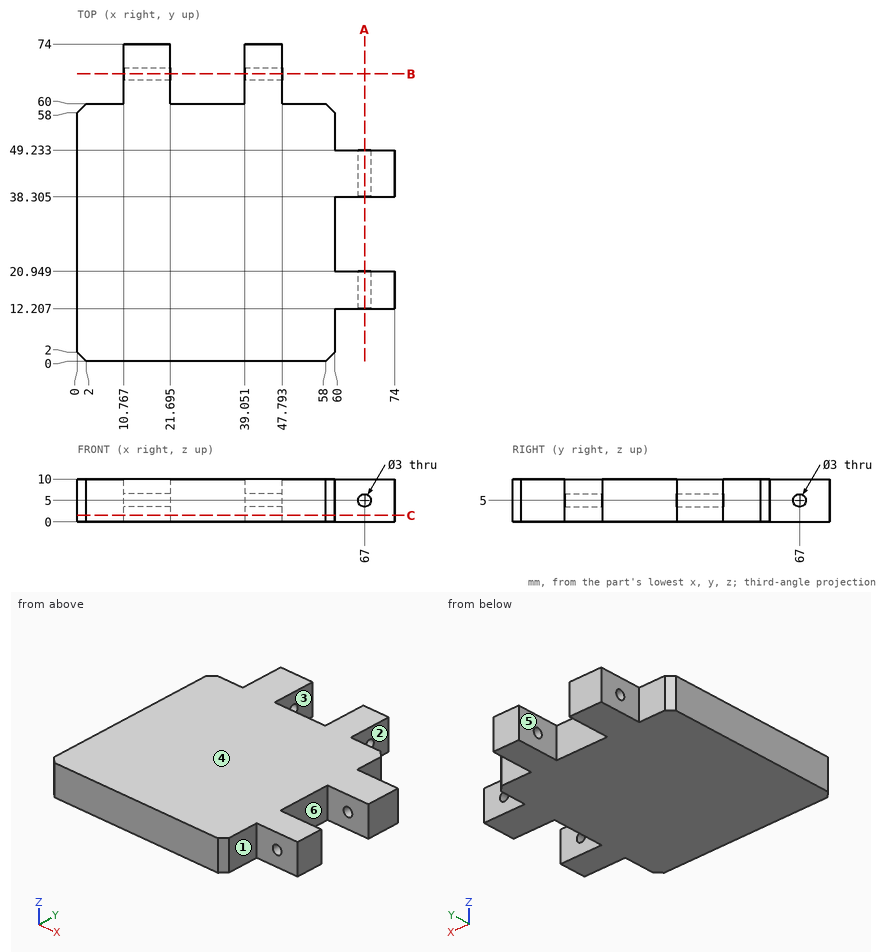
Input: dimensioned drawing with shaded views. Units: mm. Origin: part minimum x, y, z. A direction names the side the tool comes from. Coordinates: 2 decimals unless noted, no trailing zeros. Write each loop counter-clockwise with the first axis right and the second up, starting at its lowest first coordinate (ties: lowest second). Pieces come first, ordered by that corner, then holes. Notation, with made-up numbers: M 60,-8 L 101,-8 A26 ccw 101,30 Z; hole C 21,26 d7. An arc over 180 degrees is marked long. Answer as a JSON object with one key per item and string values. Group by question number.
(1) Ray query, line 1 along X through (y, z) = (44.25, 5); line 2 along Z through (x, y) = (67, 43). Return the intervals inside material, ascending. Write a range as [from, to].
(2) Section C-C on z = 1.5. Output: boundary loops of the cut face in (x, y) (1 decimal).
(3) Section B-B on y = 67. Output: boundary loops of the cut face in (x, z) (1 decimal), plus the area to 3 significant figures.
(4) Set-up query: the marked faces 1, 2 and 3. Return all of +Z, -Z, +X, -X, +Y, -Y with unobstructed straight access to the full face (end or side cutting, diameter ignored); none if empty.
(5) Section A-A on x = 67. Output: boundary loops of the cut face in (y, z) (1 decimal).
(6) Contact query for flat-ended pins moving along their axis: P1, Ø5, axis at y = 63.5, z = 5, coming from the -X side; P2, Ø3, axis at x = 51, z = 6.5, coming from the +Y side; P3, Ø2.5, axis at x = 67, z = 5, coming from the -Y side; P4, Ø3.5, axis at y = 67, z = 5, coming from the +X side. Output: stop coordinate, or through.
(7) Mould query, pull axis X, two halves, no side actions, for the marked faces 4, 5 and 6. Classes: pulls with the +X half, pulls with the -X half, needs draft (parallel to the pull), parting line crosses it, or undercut.
Result set:
{
 "1": {"line 1": "x = [0, 65.5], [68.5, 74]", "line 2": "z = [0, 3.5], [6.5, 10]"},
 "2": {"outline": "M 0,2 L 2,0 L 58,0 L 60,2 L 60,12.2 L 74,12.2 L 74,20.9 L 60,20.9 L 60,38.3 L 74,38.3 L 74,49.2 L 60,49.2 L 60,58 L 58,60 L 47.8,60 L 47.8,74 L 39.1,74 L 39.1,60 L 21.7,60 L 21.7,74 L 10.8,74 L 10.8,60 L 2,60 L 0,58 Z"},
 "3": {"outline": "M 10.8,0 L 21.7,0 L 21.7,3.5 L 10.8,3.5 Z; M 10.8,6.5 L 21.7,6.5 L 21.7,10 L 10.8,10 Z; M 39.1,0 L 47.8,0 L 47.8,3.5 L 39.1,3.5 Z; M 39.1,6.5 L 47.8,6.5 L 47.8,10 L 39.1,10 Z", "area": "138 mm2"},
 "4": {"face 1": "+Z, -Z, +X, -Y", "face 2": "+Z, -Z, +X, +Y", "face 3": "+Z, -Z, +Y"},
 "5": {"outline": "M 12.2,0 L 20.9,0 L 20.9,3.5 L 12.2,3.5 Z; M 12.2,6.5 L 20.9,6.5 L 20.9,10 L 12.2,10 Z; M 38.3,0 L 49.2,0 L 49.2,3.5 L 38.3,3.5 Z; M 38.3,6.5 L 49.2,6.5 L 49.2,10 L 38.3,10 Z"},
 "6": {"P1": "stops at x = 10.77", "P2": "stops at y = 60", "P3": "passes through", "P4": "stops at x = 47.79"},
 "7": {"face 4": "needs draft", "face 5": "undercut", "face 6": "pulls with the +X half"}
}
